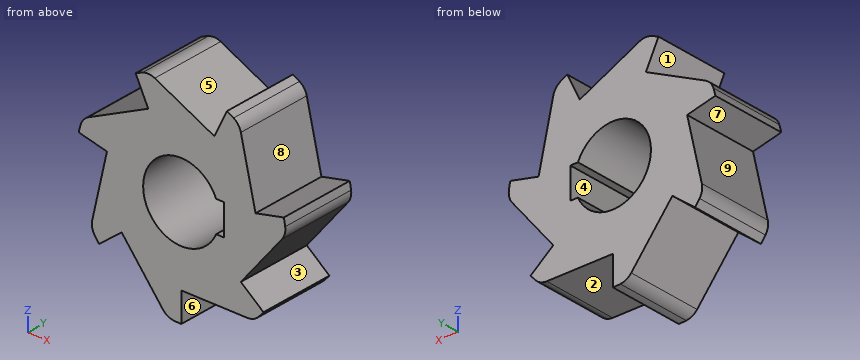
from build123d import *

# Parameters (mm, degrees)
BOSS_EXTRUDE1_DEPTH = 50


with BuildPart() as part:
    # Sketch1 → Boss-Extrude1 (new body)
    with BuildSketch(Plane(origin=(0, 0, 0), x_dir=(1, 0, 0), z_dir=(0, 1, 0))):
        with BuildLine():
            Line((0, 50), (43.370496884, 50))
            ThreePointArc((43.370496884, 50), (47.383188614, 49.159601797), (50.72142856, 46.779661017))
            ThreePointArc((50.72142856, 46.779661017), (52.367636949, 44.929173155), (53.94637229, 43.020796328))
            Line((53.94637229, 43.020796328), (39.091574123, 31.174490093))
            Line((39.091574123, 31.174490093), (66.132636632, -2.733929782))
            ThreePointArc((66.132636632, -2.733929782), (67.977459231, -6.395158214), (68.198105165, -10.488968105))
            ThreePointArc((68.198105165, -10.488968105), (67.777729639, -12.929785961), (67.270025941, -15.353944443))
            Line((67.270025941, -15.353944443), (48.746395609, -11.126046698))
            Line((48.746395609, -11.126046698), (39.095552136, -53.409154676))
            ThreePointArc((39.095552136, -53.409154676), (37.38331656, -57.134233653), (34.320217593, -59.859190308))
            ThreePointArc((34.320217593, -59.859190308), (32.149809497, -61.052352529), (29.937977999, -62.166851885))
            Line((29.937977999, -62.166851885), (21.694186956, -45.048443395))
            Line((21.694186956, -45.048443395), (-17.381280522, -63.866196751))
            ThreePointArc((-17.381280522, -63.866196751), (-21.361225962, -64.850065825), (-25.401493831, -64.154221304))
            ThreePointArc((-25.401493831, -64.154221304), (-27.687572933, -63.201252401), (-29.937977999, -62.166851885))
            Line((-29.937977999, -62.166851885), (-21.694186956, -45.048443395))
            Line((-21.694186956, -45.048443395), (-60.769654434, -26.23069004))
            ThreePointArc((-60.769654434, -26.23069004), (-64.020329644, -23.732475731), (-65.995362305, -20.13981515))
            ThreePointArc((-65.995362305, -20.13981515), (-66.675648221, -17.758320145), (-67.270025941, -15.353944443))
            Line((-67.270025941, -15.353944443), (-48.746395609, -11.126046698))
            Line((-48.746395609, -11.126046698), (-58.397239082, 31.15706128))
            ThreePointArc((-58.397239082, 31.15706128), (-58.470819328, 35.256152643), (-56.893376903, 39.040282589))
            ThreePointArc((-56.893376903, 39.040282589), (-55.455600463, 41.056989384), (-53.94637229, 43.020796328))
            Line((-53.94637229, 43.020796328), (-39.091574123, 31.174490093))
            Line((-39.091574123, 31.174490093), (-12.050511614, 65.082909967))
            ThreePointArc((-12.050511614, 65.082909967), (-8.89158947, 67.696178982), (-4.94951828, 68.822251262))
            ThreePointArc((-4.94951828, 68.822251262), (-2.476354468, 68.955548497), (0, 69))
            Line((0, 69), (0, 50))
        make_face()
        with BuildLine():
            Line((27.912878475, -10), (27.912878475, 10))
            Line((27.912878475, 10), (22.912878475, 10))
            ThreePointArc((22.912878475, 10), (-25, 0), (22.912878475, -10))
            Line((22.912878475, -10), (27.912878475, -10))
        make_face(mode=Mode.SUBTRACT)
    extrude(amount=BOSS_EXTRUDE1_DEPTH)


solid = part.part
CAD build for the part. Positions are in the model's coordinates, mm. Face numbers are marked on the shaded views. A direction names the side the tool comes from. Round coordinates to 2 decimals unless told otherwise and drop trailing zeros. Write each loop counter-clockwise with the first axis right and the second up, starting at its lowest first coordinate (ties: lowest second). Pieces come first, ordered by that corner, then holes.
(1) Probe line 1 along Z through (x, y) = (-22.5, 8.5); line 2 along Z through (x, y) = (50, 14); line 3 along X through (y, z) = (22, 0). List the from-to ranges inside material, lowest first.
(2) Mould opens along Z. For the marked faces 6, 7, 8 and 9 say: pulls with the +Z half, pulls with the -Z half, needs draft (parallel to the pull), parting line crosses it, or undercut.
(3) Drop flat-ended pins along their axis: P1, Ø1.5, axis at y = 14.5, z = 2, coming from the -X side; P2, Ø5.5, axis at x = 26, y = 34.5, coming from the -Z side; P3, Ø6, axis at x = -20, y = 9.5, coming from the -Z side. Give the stop position or say it passes through.
(4) Slice it at B-B, the plane z = -5. Write the cut outline in (x, y), and give its area (3 significant figures).
(5) 3-axis set-ups, long thin cutter, end or side, ignore diameter. For the marked faces 1, 2, 3, 4 and 5: which of +Z, -Z, +X, -X, +Y, -Y reach the whole face in a straight line?
(6) Slice it at D-D, the plane x = -43. Write the cut outline in (y, z), and give its area (3 significant figures).
(7) Slice it at C-C, the plane x = 13.5. Write the cut outline in (y, z).
From the geometry:
1. line 1: z = -51.98 to -10.9, 10.9 to 44.66, 46.72 to 64.83
1. line 2: z = -47.49 to -39.87, -17.5 to 11.41
1. line 3: x = -51.29 to -25, 27.91 to 63.95
2. face 6: needs draft
2. face 7: undercut
2. face 8: pulls with the +Z half
2. face 9: undercut
3. P1: stops at x = -51
3. P2: stops at z = -50
3. P3: stops at z = -58.88
4. outline: (-52.43, 0) - (-24.49, 0) - (-24.49, 50) - (-52.43, 50) - close; (27.91, 0) - (59.97, 0) - (59.97, 50) - (27.91, 50) - close
4. area: 3,000 mm2
5. face 1: -X, +Y, -Y
5. face 2: -Z, +X, +Y, -Y
5. face 3: +X, +Y, -Y
5. face 4: +Y, -Y
5. face 5: +Z, +Y, -Y
6. outline: (0, -34.29) - (50, -34.29) - (50, 34.79) - (0, 34.79) - close
6. area: 3,450 mm2
7. outline: (0, -50) - (50, -50) - (50, -21.04) - (0, -21.04) - close; (0, 21.04) - (50, 21.04) - (50, 48.99) - (0, 48.99) - close
